from build123d import *

# Parameters (mm, degrees)
F1_DEPTH = 3
F3_D     = 4
F4_W     = 6.5
F4_H     = 6.5
F5_DEPTH = 3
F6_R     = 2
F7_DEPTH = 3.001
F9_D     = 1


with BuildPart() as f1:
    # F0 (on Top) → F1 (new body)
    with BuildSketch(Plane.XY):
        with BuildLine():
            ThreePointArc((0, 3), (0.87868, 0.87868), (3, 0))
            Line((3, 0), (67, 0))
            ThreePointArc((67, 0), (69.12132, 0.87868), (70, 3))
            Line((70, 3), (70, 39))
            ThreePointArc((70, 39), (69.12132, 41.12132), (67, 42))
            Line((67, 42), (3, 42))
            ThreePointArc((3, 42), (0.87868, 41.12132), (0, 39))
            Line((0, 39), (0, 3))
        make_face()
    extrude(amount=F1_DEPTH)

    # F3 (through all)
    with Locations(Plane.XY.offset(3)):
        with Locations((14, 7), (24.5, 7), (35, 7), (45.5, 7), (56, 7)):
            Hole(F3_D / 2)

    # F4 (on face) → F5 (cut, through all)
    with BuildSketch(Plane.XY.offset(3)):
        with Locations((15, 21)):
            Rectangle(F4_W, F4_H)
        with Locations((55, 21)):
            Rectangle(F4_W, F4_H)
    extrude(amount=-F5_DEPTH, mode=Mode.SUBTRACT)

    # F6 (on face) → F7 (cut, through all)
    with BuildSketch(Plane.XY.offset(3)):
        with BuildLine():
            Line((57.25, 10), (12.75, 10))
            ThreePointArc((12.75, 10), (11.335786, 9.414214), (10.75, 8))
            Line((10.75, 8), (10.75, 0))
            Line((10.75, 0), (59.25, 0))
            Line((59.25, 0), (59.25, 8))
            ThreePointArc((59.25, 8), (58.664214, 9.414214), (57.25, 10))
        make_face()
        with Locations((14, 7)):
            Circle(F6_R, mode=Mode.SUBTRACT)
        with Locations((24.5, 7)):
            Circle(F6_R, mode=Mode.SUBTRACT)
        with Locations((35, 7)):
            Circle(F6_R, mode=Mode.SUBTRACT)
        with Locations((45.5, 7)):
            Circle(F6_R, mode=Mode.SUBTRACT)
        with Locations((56, 7)):
            Circle(F6_R, mode=Mode.SUBTRACT)
    extrude(amount=-F7_DEPTH, mode=Mode.SUBTRACT)

    # F9 (through all)
    with Locations(Plane.XY.offset(3)):
        with Locations((4, 38), (4, 4), (66, 4), (66, 38)):
            Hole(F9_D / 2)


solid = f1.part
Could you check a few things on this model? Use its own coordinates, in mm. A direction names the side the tool comes from. Round coordinates to 2 decimals unless told otherwise and drop trailing zeros. Write each loop counter-clockwise with the first axis right and the second up, starting at its lowest first coordinate (ties: lowest second). Pieces come first, ordered by that corner, then holes. Notation, with made-up numbers: (28.5, 45) -> (67.5, 45) arc R17 cw to (67.5, 74) -> close; hole circle Ø9 at (-11.5, 66.25). An arc over 180 degrees is marked (long way). Use a Markdown table: item, result.
1. If we section it at B-B (z = 0.45): List the corners of the cut face in (x, y) for me.
Answer key:
| item | result |
|---|---|
| outline | (0, 3) arc R3 ccw to (3, 0) -> (10.75, 0) -> (10.75, 8) arc R2 cw to (12.75, 10) -> (57.25, 10) arc R2 cw to (59.25, 8) -> (59.25, 0) -> (67, 0) arc R3 ccw to (70, 3) -> (70, 39) arc R3 ccw to (67, 42) -> (3, 42) arc R3 ccw to (0, 39) -> close; hole circle Ø1 at (4, 4); hole circle Ø1 at (4, 38); hole (11.75, 17.75) -> (18.25, 17.75) -> (18.25, 24.25) -> (11.75, 24.25) -> close; hole (51.75, 17.75) -> (58.25, 17.75) -> (58.25, 24.25) -> (51.75, 24.25) -> close; hole circle Ø1 at (66, 4); hole circle Ø1 at (66, 38) |
2. If we section it at C-C (x = 51): List the corners of the cut face in (y, z) for me.
Answer key:
| item | result |
|---|---|
| outline | (10, 0) -> (42, 0) -> (42, 3) -> (10, 3) -> close |
3. If we section it at A-A (y = 7): List the corners of the cut face in (x, z) for me, then the cut area to 3 significant figures.
Answer key:
| item | result |
|---|---|
| outline | (0, 0) -> (10.75, 0) -> (10.75, 3) -> (0, 3) -> close; (59.25, 0) -> (70, 0) -> (70, 3) -> (59.25, 3) -> close |
| area | 64.5 mm^2 |
4. Which directions (+Z, -Z, +X, -X, +Y, -Y) give clear straight access to the entire face, cutting with the end or side of a thin tool? Please do faces 5 (the face through (55, 17.75, 2)), 6 (the face through (63, 0, 1)), 7 (the face through (11.35, 9.43, 1.52)).
Answer key:
| item | result |
|---|---|
| face 5 | +Z, -Z |
| face 6 | +Z, -Z, +X, -X, -Y |
| face 7 | +Z, -Z, -Y |
5. For pin 1 Ø1.5 at (x, z) = (15.5, 1) entering from -Y, with a flat end and sliding along its axis, tell me the tip position at first contact or that it passes through.
Answer key:
| item | result |
|---|---|
| pin 1 | stops at y = 10 |
6. Please list where these lines run through material, in increasing order: probe 1 along Y at (x, z) = (4, 2.2); probe 2 along X at (y, z) = (22.5, 1); probe 3 along X at (y, z) = (38, 1.35).
Answer key:
| item | result |
|---|---|
| probe 1 | y = 0 to 3.5, 4.5 to 37.5, 38.5 to 42 |
| probe 2 | x = 0 to 11.75, 18.25 to 51.75, 58.25 to 70 |
| probe 3 | x = 0 to 3.5, 4.5 to 65.5, 66.5 to 70 |
7. We'd pull the mould along X, two halves only. Please class faces 1 (the face through (15, 24.25, 2)), 2 (the face through (35, 26, 0)), 3 (the face through (70, 21, 1)), 4 (the face through (58.25, 21, 2)): +X half, -X half, draft (parallel to the pull), parting line (faces both ways), or undercut.
Answer key:
| item | result |
|---|---|
| face 1 | undercut |
| face 2 | draft |
| face 3 | +X half |
| face 4 | undercut |
